Check sheet for the modelled part. Datum: model origin and axes. Units: mm. Face numbers are marked on the shaded views. A direction names the side the tool comes from. Round coordinates to 2 decimals unless told otherwise and drop trailing zeros. Order: outer loops, then holes, each group sorted by start corner. A loop starts at its lowest first (then second) coordinate and runs counter-clockwise, first axis right, second up. Notation, with made-up numbers: (-11, -8) -> (14, -8) arc R26 ccw to (14, 22) -> close; hole circle Ø10 at (86, 53). An arc over 180 degrees is marked (long way). Answer as CSV lines item,"result". Start each with the question number.
Autodesk Inventor part; units mm, degrees
ref_plane "Arbeitsebene1" through (0, 0, 11.5) normal (0, 0, -1) x (-1, 0, 0)
ref_plane "YZ Plane" through (0, 0, 0) normal (1, 0, 0) x (0, 1, 0)
ref_plane "XZ Plane" through (0, 0, 0) normal (0, 1, 0) x (-1, 0, 0)
sketch "Skizze1" plane through (0, 0, 0) normal (0, 0, 1) x (1, 0, 0)
  circle A0 centre (0, 0) radius 15
  dimension "d0" = 30
extrude "Extrusion1" add sketch "Skizze1" along normal blind 23
sketch "Skizze2" plane through (0, 0, 23) normal (0, 0, 1) x (1, 0, 0)
  circle A0 centre (0, 0) radius 18
  circle A1 centre (0, 0) radius 15
  dimension "d3" = 3
extrude "Extrusion2" add sketch "Skizze2" along normal blind 3 contours A0 | A1
ref_plane "Arbeitsebene1" through (0, 0, 11.5) normal (0, 0, -1) x (-1, 0, 0)
mirror "Spiegeln1" about plane through (0, 0, 11.5) normal (0, 0, -1) of "Extrusion2"
sketch "Skizze3" plane through (0, 0, 26) normal (0, 0, 1) x (1, 0, 0)
  circle A0 centre (0, 0) radius 13
  dimension "d6" = 26
extrude "Extrusion3" cut sketch "Skizze3" against normal blind 8
sketch "Skizze4" plane through (0, 0, 18) normal (0, 0, 1) x (1, 0, 0)
  circle A0 centre (0, 0) radius 11.5
  circle A1 centre (0, 0) radius 13
  dimension "d9" = 1.5
extrude "Extrusion4" cut sketch "Skizze4" against normal blind 1 contours A0
mirror "Spiegeln2" about plane through (0, 0, 11.5) normal (0, 0, -1) of "Extrusion4", "Extrusion3"
sketch "Skizze5" plane through (0, 0, 17) normal (0, 0, 1) x (1, 0, 0)
  circle A0 centre (0, 0) radius 6
  dimension "d12" = 12
extrude "Extrusion5" cut sketch "Skizze5" against normal through all
properties part number "ABS Walze" material "PC/ABS-Kunststoff"
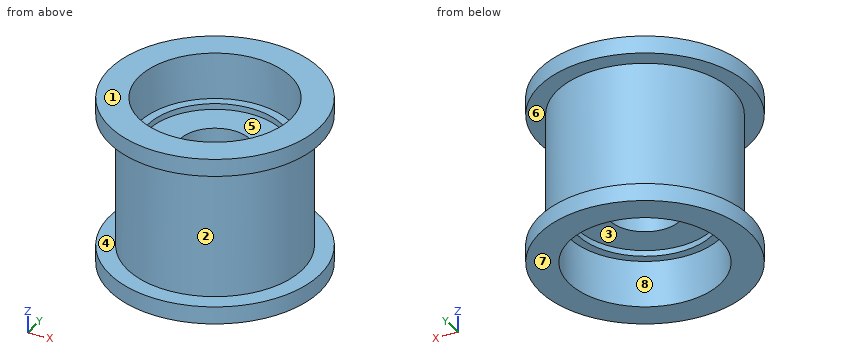
1) Material ranges on line 1 along Y through (x, z) = (0, -1); line 2 along Y through (x, z) = (0.5, 1.25); line 3 along Z through (x, y) = (0, -16), recorded low to high.
2) Access from +Z, -Z, +X, -X, +Y, -Y to the whole of each face (thin tool, end or side, straight path). Record for the marked faces 5, 6, 7 and 8.
3) Depth check by flat-ended pin: pin 1 Ø8 at (x, y) = (0.5, 3.5) entering from +Z; pin 2 Ø19 at (x, y) = (0, 0) entering from -Z; pin 3 Ø1.5 at (y, z) = (-8.5, 2) entering from +X. Enter the tip coordinate at first touch or a pass-through.
4) Mould release check, pull along Z, two halves, no side actions. Record for the marked faces 1, 2, 3 and 4: released by +Z, released by -Z, zero draft, split by the parting line, or undercut.
5) Section check D-D on y = 12.5. Record the cut outline in (x, z), then the cut area to 3 significant figures.
6) Section check C-C on z = 15.5. Record the cut outline in (x, y).
Solutions:
1,line 1,"y = -18 to -13, 13 to 18"
1,line 2,"y = -14.99 to -12.99, 12.99 to 14.99"
1,line 3,"z = -3 to 0, 23 to 26"
2,face 5,"+Z"
2,face 6,"none"
2,face 7,"-Z, +X, -X, +Y, -Y"
2,face 8,"-Z"
3,pin 1,"stops at z = 17"
3,pin 2,"stops at z = 6"
3,pin 3,"stops at x = 12.84"
4,face 1,"released by +Z"
4,face 2,"undercut"
4,face 3,"released by -Z"
4,face 4,"undercut"
5,outline,"(-12.95, -3) -> (-3.57, -3) -> (-3.57, 5) -> (3.57, 5) -> (3.57, -3) -> (12.95, -3) -> (12.95, 0) -> (8.29, 0) -> (8.29, 23) -> (12.95, 23) -> (12.95, 26) -> (3.57, 26) -> (3.57, 18) -> (-3.57, 18) -> (-3.57, 26) -> (-12.95, 26) -> (-12.95, 23) -> (-8.29, 23) -> (-8.29, 0) -> (-12.95, 0) -> close"
5,area,"423 mm^2"
6,outline,"circle Ø30 at (0, 0); hole circle Ø12 at (0, 0)"
